```python
from build123d import *

# Parameters (mm, degrees)
EXTRUDE_1_DEPTH     = 280
SKETCH_2_R          = 2.2
CUT_EXTRUDE_1_DEPTH = 280
SKETCH_3_R          = 2.2
CUT_EXTRUDE_2_DEPTH = 20


with BuildPart() as part:
    # 草图1 → 凸台-拉伸1 (new body)
    with BuildSketch(Plane(origin=(0, 0, 0), x_dir=(1, 0, 0), z_dir=(0, 1, 0))):
        Polygon((10, 0), (10, 10), (0, 10), (-10, 10), (-10, 0), (-10, -10), (0, -10), (10, -10), align=None)
        Polygon((9, 0), (9, 9), (0, 9), (-9, 9), (-9, 0), (-9, -9), (0, -9), (9, -9), align=None, mode=Mode.SUBTRACT)
    extrude(amount=-EXTRUDE_1_DEPTH)

    # 草图2 → 切除-拉伸1 (cut)
    with BuildSketch(Plane.XY.offset(10)):
        with Locations(Location((0, -40, 0), (0, 0, 180))):
            Circle(SKETCH_2_R)
        with Locations(Location((0, -80, 0), (0, 0, 180))):
            Circle(SKETCH_2_R)
        with Locations(Location((0, -120, 0), (0, 0, 180))):
            Circle(SKETCH_2_R)
        with Locations(Location((0, -180, 0), (0, 0, 180))):
            Circle(SKETCH_2_R)
        with Locations(Location((0, -220, 0), (0, 0, 180))):
            Circle(SKETCH_2_R)
        with Locations(Location((0, -260, 0), (0, 0, 180))):
            Circle(SKETCH_2_R)
    extrude(amount=-CUT_EXTRUDE_1_DEPTH, mode=Mode.SUBTRACT)

    # 草图3 → 切除-拉伸2 (cut)
    with BuildSketch(Plane(origin=(10, 0, 0), x_dir=(0, 0, -1), z_dir=(1, 0, 0))):
        with Locations((0, -60)):
            Circle(SKETCH_3_R)
        with Locations((0, -100)):
            Circle(SKETCH_3_R)
        with Locations((0, -150)):
            Circle(SKETCH_3_R)
        with Locations((0, -200)):
            Circle(SKETCH_3_R)
        with Locations((0, -240)):
            Circle(SKETCH_3_R)
    extrude(amount=-CUT_EXTRUDE_2_DEPTH, mode=Mode.SUBTRACT)


solid = part.part
```
Model file for the job. Use its own axes, mm. A direction names the side the tool comes from. Round coordinates to 2 decimals unless told otherwise and drop trailing zeros. Order: outer loops, then holes, each group sorted by start corner. A loop starts at its lowest first (then second) coordinate and runs counter-clockwise, first axis right, second up. Notation, with made-up numbers: (19, 35.5) -> (71, 35.5) arc R21 cw to (71, 44.5) -> close; hole circle Ø2 at (82.5, 88.25). An arc over 180 degrees is marked (long way). Use one line per item in the form item = value.
Item 1: Cut at A-A, the plane x = 4.75. Write the cut outline in (y, z), and give its area (3 significant figures).
Returned:
outline = (-280, -10) -> (0, -10) -> (0, -9) -> (-280, -9) -> close; (-280, 9) -> (0, 9) -> (0, 10) -> (-280, 10) -> close
area = 560 mm^2
Item 2: Flat gauge pin, fed straight in: pin 1 Ø5 at (x, z) = (1.5, 7.5) entering from -Y. Where does the tip first touch, or does it go through?
Returned:
pin_1 = -280
Item 3: Pull direction Z, two halves, no side cores. Call faces 3 (the face through (9.507, -98.145, -1.183)), 4 (the face through (-1.183, -81.855, -9.493)): released by +Z, released by -Z, zero draft, split by the parting line, or undercut.
Returned:
face_3 = undercut
face_4 = zero draft
Item 4: Tool access for faces 1 (the face through (-9.49, -147.82, 0.29)), 2 (the face through (-9, -138, 0)): list every direction of +Z, -Z, +X, -X, +Y, -Y with a clear straight run to the whole face (end or side of a thin tool).
Returned:
face_1 = +X, -X
face_2 = +Y, -Y
Item 5: Cut at B-B, the plane y = -34.5. Write the cut outline in (x, z), and give its area (3 significant figures).
Returned:
outline = (-10, -10) -> (10, -10) -> (10, 10) -> (-10, 10) -> close; hole (-9, -9) -> (9, -9) -> (9, 9) -> (-9, 9) -> close
area = 76.0 mm^2
Item 6: Drill centre lines: line 1 (Y direction, x = 9.45, z = 0); line 2 (X direction, y = -220, z = -9.7); line 3 (Z direction, x = -2.75, y = -46.5). Where is each one in solid material? Low to high.
Returned:
line_1 = -280 to -242.2, -237.8 to -202.2, -197.8 to -152.2, -147.8 to -102.2, -97.8 to -62.2, -57.8 to 0
line_2 = -10 to -2.2, 2.2 to 10
line_3 = -10 to -9, 9 to 10
